Verification items for this drawing (mm, ordinates from the low corner). A direction names the side the tool comes from. Round coordinates to 2 decimals unless told otherwise and drop trailing zeros. Loops run counter-clockwise (first coordinate to the right, second up) from the corner with the lowest first, then second, coordinate; pieces in that order, holes last. Notation, with made-up numbers: M 57,-34 L 94,-34 A27 cw 94,-1 Z; hole C -11,59.5 d1. An arc over 180 degrees is marked long. Write item = value, one per line.
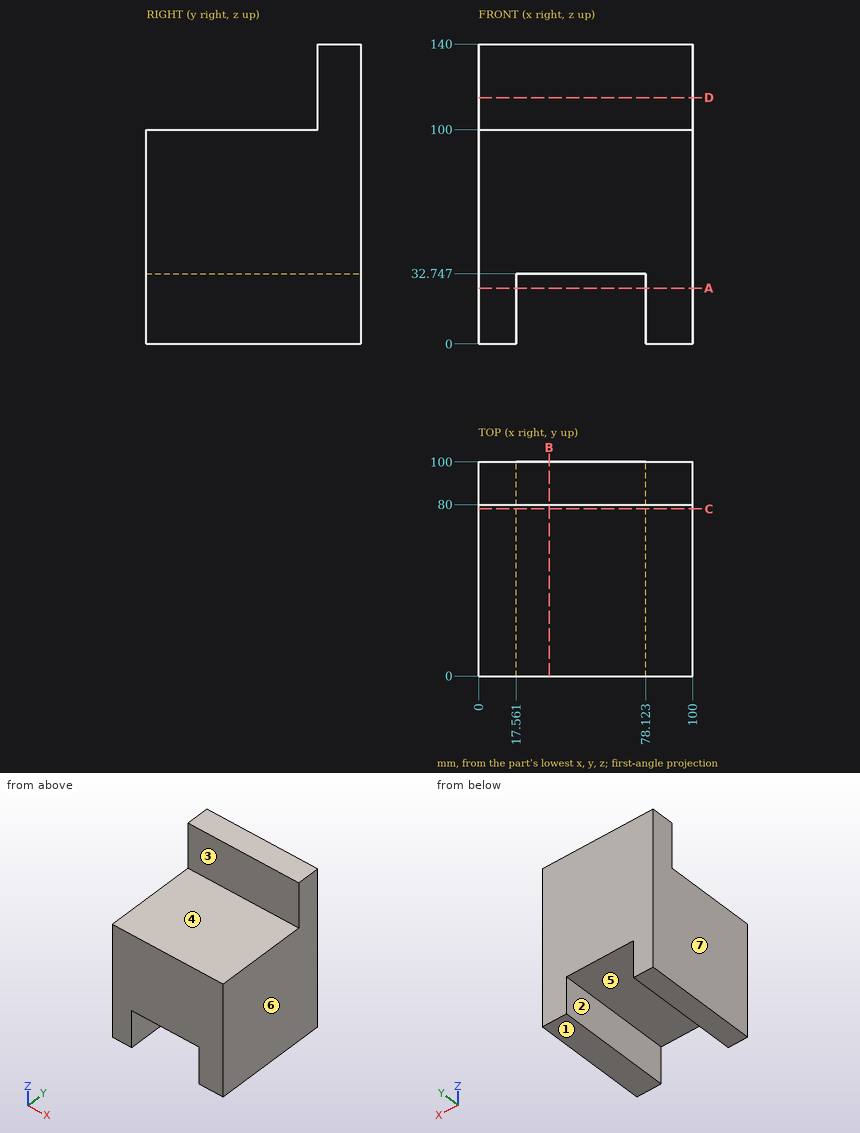
(1) Depth check by flat-ended pin: pin 1 Ø4 at (x, y) = (43, 47) entering from +Z; pin 2 Ø5 at (y, z) = (46, 23) entering from -X; pin 3 Ø2 at (x, z) = (77, 122.5) entering from -Y; pin 4 Ø8 at (x, y) = (66.5, 79.5) entering from -Z. Enter the tip coordinate at first touch or a pass-through.
Result set:
pin_1 = 100
pin_2 = 0
pin_3 = 80
pin_4 = 32.75
(2) Sectioned sample at D-D on z = 115. Record the cut outline in (x, y), then the cut area to 3 significant figures.
Result set:
outline = M 0,80 L 100,80 L 100,100 L 0,100 Z
area = 2,000 mm2
(3) Sectioned sample at B-B on x = 33. Record the cut outline in (y, z).
Result set:
outline = M 0,32.75 L 100,32.75 L 100,140 L 80,140 L 80,100 L 0,100 Z
(4) Sectioned sample at A-A on z = 26. Record the cut outline in (x, y).
Result set:
outline = M 0,0 L 17.56,0 L 17.56,100 L 0,100 Z; M 78.12,0 L 100,0 L 100,100 L 78.12,100 Z
(5) Tool access check on the marked faces 1, 2 and 3. Record the directions out of +Z, -Z, +X, -X, +Y, -Y that give a thin tool (end or side, any length) a straight path to the whole face; none if there is none.
Result set:
face_1 = -Z, +X, -X, +Y, -Y
face_2 = -Z, +Y, -Y
face_3 = +Z, +X, -X, -Y
(6) Release check for a two-part mould opening along X. For the marked faces 4, 5, 6 and 7 record: released by +X, released by -X, zero draft, split by the parting line, or undercut.
Result set:
face_4 = zero draft
face_5 = undercut
face_6 = released by +X
face_7 = released by -X
(7) Sectioned sample at C-C on y = 78. Record the cut outline in (x, z).
Result set:
outline = M 0,0 L 17.56,0 L 17.56,32.75 L 78.12,32.75 L 78.12,0 L 100,0 L 100,100 L 0,100 Z
(8) Material ranges on line 1 along X through (y, z) = (85.5, 32.5); line 2 along Z through (x, y) = (83, 44.5); line 3 along Z through (x, y) = (48.5, 34.5), recorded low to high. Write a range as from..to.
Result set:
line_1 = 0..17.56, 78.12..100
line_2 = 0..100
line_3 = 32.75..100
